Verification items for the finished model (mm, model axes). A direction names the side the tool comes from. Round coordinates to 2 decimals unless told otherwise and drop trailing zeros. Loops run counter-clockwise (first coordinate to the right, second up) from the corner with the lowest first, then second, coordinate; pieces in that order, holes last. Notation, with made-up numbers: M -11,-13.75 L 27,-13.75 A25 ccw 27,22.25 Z; hole C -5,83.25 d9. An arc over 180 degrees is marked long. Write item = value, one per line. Start each with the question number.
from build123d import *

# Parameters (mm, degrees)
F0_W     = 10
F0_H     = 10
F1_DEPTH = 25
F2_W     = 5
F2_H     = 5
F3_DEPTH = 12.5
F5_DEPTH = 12.5
F6_R     = 2
F7_DEPTH = 5


with BuildPart() as f1:
    # F0 (on Front) → F1 (new body)
    with BuildSketch(Plane.XZ):
        Rectangle(F0_W, F0_H)
    extrude(amount=F1_DEPTH)

    # F2 (on face) → F3 (cut)
    with BuildSketch(Plane.XZ.offset(25)):
        Rectangle(F2_W, F2_H)
    extrude(amount=-F3_DEPTH, mode=Mode.SUBTRACT)

    # F4 (on face) → F5 (cut)
    with BuildSketch(Plane(origin=(0, 0, 0), x_dir=(-1, 0, 0), z_dir=(0, 1, 0))):
        with BuildLine():
            Line((-2.2017970471, 1.1840987136), (2.2017970471, 1.1840987136))
            ThreePointArc((2.2017970471, 1.1840987136), (0, 2.5), (-2.2017970471, 1.1840987136))
        make_face()
        with BuildLine():
            ThreePointArc((-2.2017970471, 1.1840987136), (-0.6105355773, -2.4243032626), (2.5, 0))
            ThreePointArc((2.5, 0), (2.4243032626, 0.6105355773), (2.2017970471, 1.1840987136))
            Line((2.2017970471, 1.1840987136), (-2.2017970471, 1.1840987136))
        make_face()
        with BuildLine():
            ThreePointArc((-2.2017970471, 1.1840987136), (0, 2.5), (2.2017970471, 1.1840987136))
            Line((2.2017970471, 1.1840987136), (2.75, 1.1840987136))
            Line((2.75, 1.1840987136), (2.75, 3.1840987136))
            Line((2.75, 3.1840987136), (-2.75, 3.1840987136))
            Line((-2.75, 3.1840987136), (-2.75, 1.1840987136))
            Line((-2.75, 1.1840987136), (-2.2017970471, 1.1840987136))
        make_face()
    extrude(amount=-F5_DEPTH, mode=Mode.SUBTRACT)

    # F6 (on face) → F7 (cut)
    with BuildSketch(Plane.XY.offset(5)):
        with Locations((0, -7)):
            Circle(F6_R)
    extrude(amount=-F7_DEPTH, mode=Mode.SUBTRACT)


solid = f1.part
1. Section check D-D, the plane y = -4. Enter the section's corners in (x, z).
2. Section check A-A, the plane y = -14.75. Enter the section's corners in (x, z), and give its area (3 significant figures).
3. Gauge pin test, flat end, axial feed: P1, Ø5, axis at x = -2.5, z = -4, coming from the +Y side. Record the tip position at first contact, or that the pin passes through.
4. Section check B-B, the plane z = -2. Enter the section's corners in (x, y), and give its area (3 significant figures).
5. Section check C-C, the plane x = -1.75. Enter the section's corners in (y, z).
6. Thickness scan on line 1 (X direction, y = -7, z = 0); line 2 (Z direction, x = -1.5, y = -11); line 3 (Y direction, x = 0, z = 4.1). Record the ranges inside material, lowest first.
7. Mould release check, pull along X, two halves, no side actions. Record for faces 5 (the flat face through (0, -25, 3)), 6 (the flat face through (-2, -12.5, -2)), 7 (the flat face through (5, -12, 0)), 8 (the flat face through (-5, -12, 0)): pulls with the +X half, pulls with the -X half, needs draft (parallel to the pull), parting line crosses it, or undercut.
8. Tool access check on faces 1 (the flat face through (0, -12.5, 3)), 2 (the flat face through (0, -19, 2.5)), 3 (the flat face through (0, -19, -2.5)), 4 (the cylindrical face through (1.908, -6.399, 4.105)). Record the directions out of +Z, -Z, +X, -X, +Y, -Y that give a thin tool (end or side, any length) a straight path to the whole face; none if there is none.
Computed values:
q1.outline = M -5,-5 L 5,-5 L 5,5 L -5,5 Z; hole M -2.75,1.18 L -2.2,1.18 A2.5 ccw long 2.2,1.18 L 2.75,1.18 L 2.75,3.18 L -2.75,3.18 Z
q2.outline = M -5,-5 L 5,-5 L 5,5 L -5,5 Z; hole M -2.5,-2.5 L 2.5,-2.5 L 2.5,2.5 L -2.5,2.5 Z
q2.area = 75.0 mm2
q3.P1 = 0
q4.outline = M -5,-25 L -2.5,-25 L -2.5,-12.5 L -1.5,-12.5 L -1.5,0 L -5,0 Z; M 1.5,-12.5 L 2.5,-12.5 L 2.5,-25 L 5,-25 L 5,0 L 1.5,0 Z
q4.area = 150 mm2
q5.outline = M -25,-5 L 0,-5 L 0,-1.79 L -12.5,-1.79 L -12.5,-2.5 L -25,-2.5 Z; M -25,2.5 L -12.5,2.5 L -12.5,3.18 L -7.97,3.18 L -7.97,5 L -25,5 Z; M -6.03,3.18 L 0,3.18 L 0,5 L -6.03,5 Z
q6.line_1 = -5 to -2.5, 2.5 to 5
q6.line_2 = -5 to -2, 3.18 to 5
q6.line_3 = -25 to -9, -5 to 0
q7.face_5 = needs draft
q7.face_6 = undercut
q7.face_7 = pulls with the +X half
q7.face_8 = pulls with the -X half
q8.face_1 = +Y
q8.face_2 = +Y, -Y
q8.face_3 = -Y
q8.face_4 = +Z
